```python
from build123d import *

# Parameters (mm, degrees)
BOSS_EXTRUDE1_DEPTH = 2000


with BuildPart() as part:
    # Sketch1 → Boss-Extrude1 (new body)
    with BuildSketch(Plane.XY):
        with BuildLine():
            Line((-15.5, -20), (-5, -20))
            Line((-5, -20), (-5, -10))
            Line((-5, -10), (5, -10))
            Line((5, -10), (5, -20))
            Line((5, -20), (15.5, -20))
            ThreePointArc((15.5, -20), (18.681980515, -18.681980515), (20, -15.5))
            Line((20, -15.5), (20, 15.5))
            ThreePointArc((20, 15.5), (18.681980515, 18.681980515), (15.5, 20))
            Line((15.5, 20), (-8, 20))
            Line((-8, 20), (-8, 10))
            Line((-8, 10), (-15, 10))
            Line((-15, 10), (-15, 20))
            Line((-15, 20), (-15.5, 20))
            ThreePointArc((-15.5, 20), (-18.681980515, 18.681980515), (-20, 15.5))
            Line((-20, 15.5), (-20, -15.5))
            ThreePointArc((-20, -15.5), (-18.681980515, -18.681980515), (-15.5, -20))
        make_face()
    extrude(amount=BOSS_EXTRUDE1_DEPTH)


solid = part.part
```
Geometry: final body of the model. Coordinates: model frame, mm. Round coordinates to 2 decimals unless told otherwise and drop trailing zeros. Write each loop counter-clockwise with the first axis right and the second up, starting at its lowest first coordinate (ties: lowest second). Pieces come first, ordered by that corner, then holes. Notation, with made-up numbers: M 18.5,53 L 67.5,53 A35 ccw 67.5,86 Z; hole C 49,31 d8. An arc over 180 degrees is marked long. Answer in a Markdown table with one row per item. Add a question column.
(1) Ray query, L1, parallel to X at y = 15.5, z = 1003; L2, parallel to X at y = -12.5, z = 721.5; L3, parallel to Y at x = -4.5, z = 123.5. Return the intervals inside material, ascending.
(2) Contact query for flat-ended pins moving along their axis: pin 1 (3 mm diameter, centred on x = -10.5, z = 1552.5, fed in from +Y); pin 2 (8 mm diameter, centred on x = 0.5, z = 1147, fed in from -Y). Output: stop coordinate, or through.
(3) Cut plane A-A, the plane z = 532. Return the cut outline in (x, y).
Established:
| question | item | result |
|---|---|---|
| 1 | L1 | -20 to -15, -8 to 20 |
| 1 | L2 | -20 to -5, 5 to 20 |
| 1 | L3 | -10 to 20 |
| 2 | pin 1 | y = 10 |
| 2 | pin 2 | y = -10 |
| 3 | outline | M -20,-15.5 A4.5 ccw -15.5,-20 L -5,-20 L -5,-10 L 5,-10 L 5,-20 L 15.5,-20 A4.5 ccw 20,-15.5 L 20,15.5 A4.5 ccw 15.5,20 L -8,20 L -8,10 L -15,10 L -15,20 L -15.5,20 A4.5 ccw -20,15.5 Z |
